Part model, mm, in its own coordinate system. A direction names the side the tool comes from. Give positions to 0.01 mm unless a question says otherwise; leave off trailing zeros. Write each loop counter-clockwise with the first axis right and the second up, starting at its lowest first coordinate (ties: lowest second). Pieces come first, ordered by that corner, then holes. Notation, with made-up numbers: M -35.5,4 L 14.5,4 A29 cw 14.5,29 Z; hole C 53.25,15 d1. An arc over 180 degrees is marked long. Answer as CSV lines item,"result". Start each with the question number.
1) Pin check, flat tips, straight feed: pin 1 Ø0.5 at (x, z) = (0.5, 0) entering from +Y; pin 2 Ø2 at (x, z) = (1, 0) entering from +Y. Stop position of each tip, or through.
2) Tool access for faces 1 (the flat face through (0, 43, 0.5)), 2 (the flat face through (0, 0, 0)): list every direction of +Z, -Z, +X, -X, +Y, -Y with a clear straight run to the whole face (end or side of a thin tool).
3) Slice it at D-D, the plane z = 0. Give the cut face in (x, y), plus the area to 3 significant figures.
4) Slice it at C-C, the plane y = 19.5. Give the cut face in (x, z), plus the area to 3 significant figures.
5) Wall check: line 1 along Z through (x, y) = (-0.1, 31.5); line 2 along X through (y, z) = (4.5, -0.55); line 3 along Y through (x, z) = (-0.55, 0.15). Give the ranges that are in metal, low to high. Write a range as from..to.
6) Mould opens along Z. For faces 3 (the cylindrical face through (-2.54, 22.18, 1.05)), 4 (the flat face through (0, 45, -1)), 5 (the flat face through (0, 40, 0)) say: pulls with the +Z half, pulls with the -Z half, needs draft (parallel to the pull), parting line crosses it, or undercut.
7) Slice it at A-A, the plane x = 0. Give the cut face in (y, z), plus the area to 4 significant figures.
8) Slice it at B-B, the plane z = -1.65. Give the cut face in (x, y).
Autodesk Inventor part; units mm, degrees
ref_plane "YZ Plane" through (0, 0, 0) normal (1, 0, 0) x (0, 1, 0)
ref_plane "XZ Plane" through (0, 0, 0) normal (0, 1, 0) x (-1, 0, 0)
ref_plane "XY Plane" through (0, 0, 0) normal (0, 0, 1) x (1, 0, 0)
sketch "Sketch1" plane through (0, 0, 0) normal (0, 1, 0) x (-1, 0, 0)
  circle A0 centre (0, 0) radius 2.75
  dimension "d0" = 5.5
extrude "Extrusion1" add sketch "Sketch1" along normal blind 45
sketch "Sketch2" plane through (0, 45, 0) normal (0, 1, 0) x (1, 0, 0)
  line L0 (3.6897, -0.5) -> (3.6897, 0.5)
  line L1 (3.6897, 0.5) -> (-3.6897, 0.5)
  line L2 (-3.6897, 0.5) -> (-3.6897, -0.5)
  line L3 (-3.6897, -0.5) -> (3.6897, -0.5)
  line L4 (3.6897, -0.5) -> (-3.6897, 0.5) construction
  line L5 (3.6897, 0.5) -> (-3.6897, -0.5) construction
  point P0 (0, 0)
  dimension "d3" = 1
extrude "Extrusion2" cut sketch "Sketch2" against normal blind 5
properties part number "Solenoid Interior"
Found:
1,pin 1,"y = 40"
1,pin 2,"y = 45"
2,face 1,"+X, -X, +Y"
2,face 2,"+Z, -Z, +X, -X, -Y"
3,outline,"M -2.75,0 L 2.75,0 L 2.75,40 L -2.75,40 Z"
3,area,"220 mm²"
4,outline,"C 0,0 d5.5"
4,area,"23.8 mm²"
5,line 1,"-2.75..2.75"
5,line 2,"-2.69..2.69"
5,line 3,"0..40"
6,face 3,"parting line crosses it"
6,face 4,"needs draft"
6,face 5,"undercut"
7,outline,"M 0,-2.75 L 45,-2.75 L 45,-0.5 L 40,-0.5 L 40,0.5 L 45,0.5 L 45,2.75 L 0,2.75 Z"
7,area,"242.5 mm²"
8,outline,"M -2.2,0 L 2.2,0 L 2.2,45 L -2.2,45 Z"
